from build123d import *

# Parameters (mm, degrees)
SKETCH1_W           = 33.5
SKETCH1_H           = 33.5
SKETCH1_W_2         = 29.5
SKETCH1_H_2         = 29.5
BOSS_EXTRUDE1_DEPTH = 39.5
SKETCH2_W           = 29.5
SKETCH2_H           = 29.5
BOSS_EXTRUDE2_DEPTH = 3
FILLET_1_R          = 2
FILLET_2_R          = 2
FILLET_3_R          = 1


with BuildPart() as part:
    # Sketch1 → Boss-Extrude1 (new body)
    with BuildSketch(Plane(origin=(0, 0, 0), x_dir=(1, 0, 0), z_dir=(0, 1, 0))):
        with Locations((16.75, 16.75)):
            Rectangle(SKETCH1_W, SKETCH1_H)
        with Locations((16.75, 16.75)):
            Rectangle(SKETCH1_W_2, SKETCH1_H_2, mode=Mode.SUBTRACT)
    extrude(amount=BOSS_EXTRUDE1_DEPTH)

    # Sketch2 → Boss-Extrude2 (add)
    with BuildSketch(Plane.XZ):
        with Locations((16.75, -16.75)):
            Rectangle(SKETCH2_W, SKETCH2_H)
    extrude(amount=-BOSS_EXTRUDE2_DEPTH)

    # Скругление1
    fillet_1_edges = [part.edges().sort_by_distance(p)[0] for p in [
        (0, 19.75, -33.5),
        (33.5, 19.75, -33.5),
        (33.5, 19.75, 0),
        (0, 19.75, 0),
    ]]
    fillet(fillet_1_edges, radius=FILLET_1_R)

    # Скругление2
    fillet_2_edges = [part.edges().sort_by_distance(p)[0] for p in [
        (0, 0, -16.75),
        (16.75, 0, -33.5),
        (33.5, 0, -16.75),
        (16.75, 0, 0),
        (32.914213562, 0, -0.585786438),
        (32.914213562, 0, -32.914213562),
        (0.585786438, 0, -0.585786438),
        (0.585786438, 0, -32.914213562),
    ]]
    fillet(fillet_2_edges, radius=FILLET_2_R)

    # Скругление3
    fillet_3_edges = [part.edges().sort_by_distance(p)[0] for p in [
        (2, 21.25, -31.5),
        (2, 21.25, -2),
        (31.5, 21.25, -2),
        (31.5, 21.25, -31.5),
        (2, 39.5, -16.75),
        (16.75, 39.5, -2),
        (31.5, 39.5, -16.75),
        (16.75, 39.5, -31.5),
        (16.75, 3, -31.5),
        (2, 3, -16.75),
        (16.75, 3, -2),
        (31.5, 3, -16.75),
    ]]
    fillet(fillet_3_edges, radius=FILLET_3_R)


solid = part.part
Verification items for the finished model (mm, model axes). A direction names the side the tool comes from. Coordinates: 2 decimals unless noted, no trailing zeros. Order: outer loops, then holes, each group sorted by start corner. A loop starts at its lowest first (then second) coordinate and runs counter-clockwise, first axis right, second up. Notation, with made-up numbers: M 79.25,33 L 105.25,33 A15 ccw 105.25,62 Z; hole C -25,52 d2. An arc over 180 degrees is marked long. Return JSON: item names as keys, results as strings.
1) Cross-section at A-A, the plane y = 24.5. Record the boundary of the cut face in (x, z).
Answer list:
{"outline": "M 0,-31.5 A2 ccw 2,-33.5 L 31.5,-33.5 A2 ccw 33.5,-31.5 L 33.5,-2 A2 ccw 31.5,0 L 2,0 A2 ccw 0,-2 Z; hole M 2,-30.5 A1 ccw 3,-31.5 L 30.5,-31.5 A1 ccw 31.5,-30.5 L 31.5,-3 A1 ccw 30.5,-2 L 3,-2 A1 ccw 2,-3 Z"}
2) Thickness scan on L1, parallel to Z at x = 11, y = 37; L2, parallel to X at y = 12, z = -25.5; L3, parallel to Y at x = 22.5, z = -24. Record the ranges inside material, lowest first. Write a range as [from, to].
Answer list:
{"L1": "[-33.5, -31.5], [-2, 0]", "L2": "[0, 2], [31.5, 33.5]", "L3": "[0, 3]"}
3) Gauge pin test, flat ends, axial feed: pin 1 (4 mm diameter, centred on x = 3.5, z = -18, fed in from +Y); pin 2 (14 mm diameter, centred on x = 21.5, z = -19, fed in from +Y). Record the tip position at first contact, or that the pin passes through.
Answer list:
{"pin 1": "y = 39.37", "pin 2": "y = 3"}
4) Release check for a two-part mould opening along Z. For faces 3 (the flat face through (33.5, 20, -17)), 4 (the flat face through (17, 20, -33.5)), 5 (the cylindrical face through (0.57, 21.01, -0.6)), 6 (the cylindrical face through (16.943, 39.215, -1.699)) record: +Z half, -Z half, draft (parallel to the pull), parting line (faces both ways), or undercut.
Answer list:
{"face 3": "draft", "face 4": "-Z half", "face 5": "+Z half", "face 6": "undercut"}
5) Access from +Z, -Z, +X, -X, +Y, -Y to the whole of each face (thin tool, end or side, straight path). Record for faces 1 (the cylindrical face through (31.215, 3.301, -16.557)), 2 (the cylindrical face through (32.9, 21.01, -0.57)).
Answer list:
{"face 1": "+Y", "face 2": "+Z, +X, +Y, -Y"}
6) Cross-section at B-B, the plane x = 10. Record the boundary of the cut face in (y, z), and give its area (3 significant figures).
Answer list:
{"outline": "M 0,-31.5 A2 ccw 2,-33.5 L 39.5,-33.5 L 39.5,-32.5 A1 ccw 38.5,-31.5 L 4,-31.5 A1 cw 3,-30.5 L 3,-3 A1 cw 4,-2 L 38.5,-2 A1 ccw 39.5,-1 L 39.5,0 L 2,0 A2 ccw 0,-2 Z", "area": "245 mm2"}
7) Cross-section at C-C, the plane z = -28. Record the boundary of the cut face in (x, y), and give its area (3 significant figures).
Answer list:
{"outline": "M 0,2 A2 ccw 2,0 L 31.5,0 A2 ccw 33.5,2 L 33.5,39.5 L 32.5,39.5 A1 ccw 31.5,38.5 L 31.5,4 A1 cw 30.5,3 L 3,3 A1 cw 2,4 L 2,38.5 A1 ccw 1,39.5 L 0,39.5 Z", "area": "245 mm2"}
